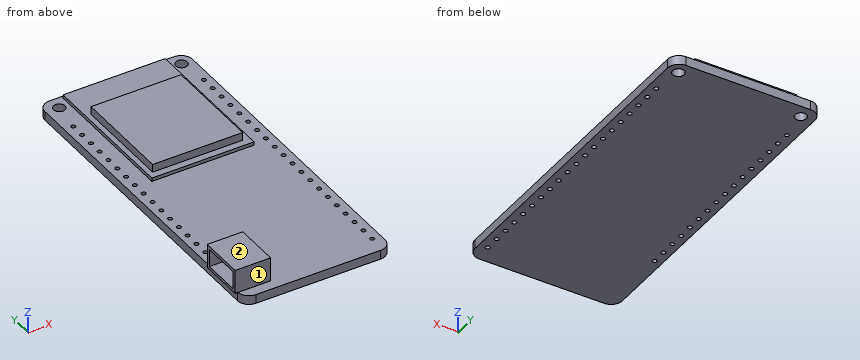
```python
from build123d import *

# Parameters (mm, degrees)
ESQUISSE3_W             = 15.791637012
ESQUISSE3_H             = 17.590684267
BOSS_EXTRU_1_DEPTH      = 2
ESQUISSE2_W             = 17.933359934
ESQUISSE2_H             = 25.329443091
BOSS_EXTRU_2_DEPTH      = 0.6
ESQUISSE4_W             = 6.231089561
ESQUISSE4_H             = 7.934254041
BOSS_EXTRU_3_DEPTH      = 4.2
ESQUISSE5_W             = 3.122951255
ESQUISSE5_H             = 6.687685859
ENL_V_MAT_EXTRU_1_DEPTH = 4.2
ESQUISSE1_R             = 1.007769755
ESQUISSE1_R_2           = 1.015003651
ESQUISSE1_R_3           = 0.379085232
ESQUISSE1_R_4           = 0.384809787
BOSS_EXTRU_5_DEPTH      = 1.6


with BuildPart() as part:
    # Esquisse3 → Boss.-Extru.1 (new body)
    with BuildSketch(Plane.XY):
        with Locations((22.462662563, 538.851133679)):
            Rectangle(ESQUISSE3_W, ESQUISSE3_H)
    extrude(amount=BOSS_EXTRU_1_DEPTH)

    # Esquisse2 → Boss.-Extru.2 (add)
    with BuildSketch(Plane.XY):
        with Locations((22.619722244, 541.464035644)):
            Rectangle(ESQUISSE2_W, ESQUISSE2_H)
    extrude(amount=BOSS_EXTRU_2_DEPTH)



with BuildPart() as body_2:
    # Esquisse4 → Boss.-Extru.3 (new body)
    with BuildSketch(Plane.XY):
        with Locations((12.149458307, 501.526955697)):
            Rectangle(ESQUISSE4_W, ESQUISSE4_H)
    extrude(amount=BOSS_EXTRU_3_DEPTH)

    # Esquisse5 → Enlèv. mat.-Extru.1 (cut)
    with BuildSketch(Plane.ZY.offset(-9.033913526)):
        with Locations((2.075345186, 501.536635321)):
            Rectangle(ESQUISSE5_W, ESQUISSE5_H)
    extrude(amount=-ENL_V_MAT_EXTRU_1_DEPTH, mode=Mode.SUBTRACT)


with BuildPart() as part_1:
    add(part.part)

    add(body_2.part)  # Boss.-Extru.5 merges body 2
    # Esquisse1 → Boss.-Extru.5 (add)
    with BuildSketch(Plane.XY):
        with BuildLine():
            Line((11.53160478, 495.667835537), (33.413782108, 495.667835537))
            ThreePointArc((33.413782108, 495.667835537), (34.82799567, 496.253621975), (35.413782108, 497.667835537))
            Line((35.413782108, 497.667835537), (35.413782108, 552.585869124))
            ThreePointArc((35.413782108, 552.585869124), (34.82799567, 554.000082687), (33.413782108, 554.585869124))
            Line((33.413782108, 554.585869124), (11.53160478, 554.585869124))
            ThreePointArc((11.53160478, 554.585869124), (10.117391217, 554.000082687), (9.53160478, 552.585869124))
            Line((9.53160478, 552.585869124), (9.53160478, 497.667835537))
            ThreePointArc((9.53160478, 497.667835537), (10.117391217, 496.253621975), (11.53160478, 495.667835537))
        make_face()
        with Locations((11.851858825, 552.281521948)):
            Circle(ESQUISSE1_R, mode=Mode.SUBTRACT)
        with Locations((33.388345227, 552.400453993)):
            Circle(ESQUISSE1_R_2, mode=Mode.SUBTRACT)
        with Locations((11.106340619, 547.074143577)):
            Circle(ESQUISSE1_R_3, mode=Mode.SUBTRACT)
        with Locations((11.088253425, 544.534207977)):
            Circle(ESQUISSE1_R_3, mode=Mode.SUBTRACT)
        with Locations((11.070166231, 541.994272377)):
            Circle(ESQUISSE1_R_3, mode=Mode.SUBTRACT)
        with Locations((11.052079036, 539.454336777)):
            Circle(ESQUISSE1_R_3, mode=Mode.SUBTRACT)
        with Locations((11.033991842, 536.914401176)):
            Circle(ESQUISSE1_R_3, mode=Mode.SUBTRACT)
        with Locations((11.015904648, 534.374465576)):
            Circle(ESQUISSE1_R_3, mode=Mode.SUBTRACT)
        with Locations((10.997817454, 531.834529976)):
            Circle(ESQUISSE1_R_3, mode=Mode.SUBTRACT)
        with Locations((10.979730259, 529.294594376)):
            Circle(ESQUISSE1_R_3, mode=Mode.SUBTRACT)
        with Locations((10.961643065, 526.754658775)):
            Circle(ESQUISSE1_R_3, mode=Mode.SUBTRACT)
        with Locations((10.943555871, 524.214723175)):
            Circle(ESQUISSE1_R_3, mode=Mode.SUBTRACT)
        with Locations((10.925468676, 521.674787575)):
            Circle(ESQUISSE1_R_3, mode=Mode.SUBTRACT)
        with Locations((10.907381482, 519.134851975)):
            Circle(ESQUISSE1_R_3, mode=Mode.SUBTRACT)
        with Locations((10.889294288, 516.594916374)):
            Circle(ESQUISSE1_R_3, mode=Mode.SUBTRACT)
        with Locations((10.871207093, 514.054980774)):
            Circle(ESQUISSE1_R_3, mode=Mode.SUBTRACT)
        with Locations((10.853119899, 511.515045174)):
            Circle(ESQUISSE1_R_3, mode=Mode.SUBTRACT)
        with Locations((10.835032705, 508.975109574)):
            Circle(ESQUISSE1_R_3, mode=Mode.SUBTRACT)
        with Locations((34.05821266, 547.138652956)):
            Circle(ESQUISSE1_R_4, mode=Mode.SUBTRACT)
        with Locations((34.051054062, 544.598663044)):
            Circle(ESQUISSE1_R_4, mode=Mode.SUBTRACT)
        with Locations((34.043895464, 542.058673131)):
            Circle(ESQUISSE1_R_4, mode=Mode.SUBTRACT)
        with Locations((34.036736867, 539.518683219)):
            Circle(ESQUISSE1_R_4, mode=Mode.SUBTRACT)
        with Locations((34.029578269, 536.978693307)):
            Circle(ESQUISSE1_R_4, mode=Mode.SUBTRACT)
        with Locations((34.022419671, 534.438703395)):
            Circle(ESQUISSE1_R_4, mode=Mode.SUBTRACT)
        with Locations((34.015261074, 531.898713482)):
            Circle(ESQUISSE1_R_4, mode=Mode.SUBTRACT)
        with Locations((34.008102476, 529.35872357)):
            Circle(ESQUISSE1_R_4, mode=Mode.SUBTRACT)
        with Locations((34.000943878, 526.818733658)):
            Circle(ESQUISSE1_R_4, mode=Mode.SUBTRACT)
        with Locations((33.993785281, 524.278743745)):
            Circle(ESQUISSE1_R_4, mode=Mode.SUBTRACT)
        with Locations((33.986626683, 521.738753833)):
            Circle(ESQUISSE1_R_4, mode=Mode.SUBTRACT)
        with Locations((33.979468085, 519.198763921)):
            Circle(ESQUISSE1_R_4, mode=Mode.SUBTRACT)
        with Locations((33.972309488, 516.658774009)):
            Circle(ESQUISSE1_R_4, mode=Mode.SUBTRACT)
        with Locations((33.96515089, 514.118784096)):
            Circle(ESQUISSE1_R_4, mode=Mode.SUBTRACT)
        with Locations((33.957992292, 511.578794184)):
            Circle(ESQUISSE1_R_4, mode=Mode.SUBTRACT)
        with Locations((33.950833695, 509.038804272)):
            Circle(ESQUISSE1_R_4, mode=Mode.SUBTRACT)
        with Locations((33.943675097, 506.498814359)):
            Circle(ESQUISSE1_R_4, mode=Mode.SUBTRACT)
        with Locations((33.9365165, 503.958824447)):
            Circle(ESQUISSE1_R_4, mode=Mode.SUBTRACT)
        with Locations((33.929357902, 501.418834535)):
            Circle(ESQUISSE1_R_4, mode=Mode.SUBTRACT)
        with Locations((33.922199304, 498.878844623)):
            Circle(ESQUISSE1_R_4, mode=Mode.SUBTRACT)
    extrude(amount=-BOSS_EXTRU_5_DEPTH)


solid = part_1.part
```
The listing builds one solid part. Answer for the finished solid, in the listing's coordinates (mm). Face numbers are marked on the shaded views. A direction names the side the tool comes from. Give positions to 0.01 mm unless a question says otherwise; leave off trailing zeros. Loops run counter-clockwise (first coordinate to the right, second up) from the corner with the lowest first, then second, coordinate; pieces in that order, holes last. Notation, with made-up numbers: M -35.75,23.5 L -16.75,23.5 A15 ccw -16.75,35.5 Z; hole C 13,24 d11. An arc over 180 degrees is marked long. One line per item, written item: value.
Q1. Flat-ended cylindrical pins translate along their axes: P1, Ø2.5, axis at x = 11.85, y = 552.28, coming from the -Z side; P2, Ø2, axis at y = 501, z = 2, coming from the +X side (3 decimals); P3, Ø1.1, axis at y = 536.5, z = 1, coming from the +X side; P4, Ø2.5, axis at x = 33.39, y = 552.4, coming from the +Z side. Find the tip coordinate at first contact, or state that the pin passes through.
Working result:
P1: stops at z = -1.6
P2: stops at x = 15.265
P3: stops at x = 31.59
P4: stops at z = 0
Q2. Find the intervals of material crossed by line 1 (X direction, y = 521.5, z = -0.4); line 2 (Y direction, x = 10.25, z = 0.95); line 3 (Z direction, x = 22.5, y = 512.5), in increasing order. Write a range as from..to.
Working result:
line 1: x = 9.53..10.59, 11.26..33.68, 34.29..35.41
line 2: y = 497.56..498.19, 504.88..505.49
line 3: z = -1.6..0
Q3. A cutting plane is placed at A-A on z = 1.3. Determine the outline of the cut face in (x, y) (3 decimals).
Working result:
outline: M 9.034,497.56 L 15.265,497.56 L 15.265,505.494 L 9.034,505.494 L 9.034,504.88 L 13.234,504.88 L 13.234,498.193 L 9.034,498.193 Z; M 14.567,530.056 L 30.358,530.056 L 30.358,547.646 L 14.567,547.646 Z
Q4. For the marked faces 1 and 2, determine the directions among +Z, -Z, +X, -X, +Y, -Y from which every point of the face is accessible in a straight line to the end or side of a thin tool.
Working result:
face 1: +Z, +X, -X, -Y
face 2: +Z, +X, -X, +Y, -Y
Q5. A cutting plane is placed at C-C on y = 546. Determine the outline of the cut face in (x, z), then the cut area to 3 significant figures.
Working result:
outline: M 9.53,-1.6 L 35.41,-1.6 L 35.41,0 L 31.59,0 L 31.59,0.6 L 30.36,0.6 L 30.36,2 L 14.57,2 L 14.57,0.6 L 13.65,0.6 L 13.65,0 L 9.53,0 Z
area: 74.3 mm^2
Q6. A cutting plane is placed at B-B on x = 23.25. Determine the outline of the cut face in (y, z).
Working result:
outline: M 495.67,-1.6 L 554.59,-1.6 L 554.59,0 L 554.13,0 L 554.13,0.6 L 547.65,0.6 L 547.65,2 L 530.06,2 L 530.06,0.6 L 528.8,0.6 L 528.8,0 L 495.67,0 Z
Q7. A cutting plane is placed at D-D on z = -1.05. Give the number of separate pieces and of enclosed holes in the cut face, then the cut area to 3 significant figures.
Working result:
separate pieces: 1
enclosed holes: 38
area: 1,500 mm^2
